from build123d import *

# Parameters (mm, degrees)
F0_W     = 31.75
F0_H     = 16.51
F0_W_2   = 26.67
F0_H_2   = 11.43
F1_DEPTH = 304.8
F2_SIZE  = 1.27
F3_SIZE  = 1.27
F5_D     = 12.7
F5_DEPTH = 25.4


with BuildPart() as f1:
    # F0 (on Top) → F1 (new body)
    with BuildSketch(Plane.XY):
        Rectangle(F0_W, F0_H)
        Rectangle(F0_W_2, F0_H_2, mode=Mode.SUBTRACT)
    extrude(amount=F1_DEPTH)

    # F2
    f2_edges = [f1.edges().sort_by_distance(p)[0] for p in [
        (0, 5.715, 304.8),
        (-13.335, 0, 304.8),
        (0, -5.715, 304.8),
        (13.335, 0, 304.8),
    ]]
    chamfer(f2_edges, length=F2_SIZE)

    # F3
    f3_edges = [f1.edges().sort_by_distance(p)[0] for p in [
        (13.335, 0, 0),
        (0, 5.715, 0),
        (-13.335, 0, 0),
        (0, -5.715, 0),
    ]]
    chamfer(f3_edges, length=F3_SIZE)

    # F5
    with Locations(Plane.XZ.offset(8.255)):
        with Locations((0, 152.39365), (0, 247.65), (0.458365, 57.15)):
            Hole(F5_D / 2, depth=F5_DEPTH)


solid = f1.part
The listing builds one solid part. Answer for the finished solid, in the listing's coordinates (mm). A direction names the side the tool comes from. Give positions to 0.01 mm unless a question says otherwise; leave off trailing zeros. Write each loop counter-clockwise with the first axis right and the second up, starting at its lowest first coordinate (ties: lowest second). Pieces come first, ordered by that corner, then holes. Notation, with made-up numbers: (-18.5, -32.5) - (36.5, -32.5) arc R12 cw to (36.5, -10.5) - close; hole circle Ø3 at (62.5, 74.5). An arc over 180 degrees is marked (long way). Use a Markdown table: item, result.
1. A tool of negligible diameter and unlimited length cuts with its end or side. For faces 1 (the flat face through (-9, 5.715, 150)), 2 (the cylindrical face through (1.38, 7, 241.45)), from which of +Z, -Z, +X, -X, +Y, -Y can it reach the whole face along a straight path? Write none if from no direction.
Values follow:
| item | result |
|---|---|
| face 1 | +Z, -Z |
| face 2 | +Y, -Y |
2. Section C-C on z = 79.5 is taken. Write down the section's boundary in (x, y) (3 decimals).
Values follow:
| item | result |
|---|---|
| outline | (-15.875, -8.255) - (15.875, -8.255) - (15.875, 8.255) - (-15.875, 8.255) - close; hole (-13.335, -5.715) - (13.335, -5.715) - (13.335, 5.715) - (-13.335, 5.715) - close |
3. For a pull along X with two mould halves and no side action, classify faces 3 (the flat face through (-1.3, -7.3, 0)), 4 (the flat face through (-9, -5.715, 150)), 5 (the flat face through (15.875, 0, 150)), 6 (the flat face through (-15.875, 0, 150)) as released by +X, released by -X, zero draft, split by the parting line, or undercut.
Values follow:
| item | result |
|---|---|
| face 3 | zero draft |
| face 4 | undercut |
| face 5 | released by +X |
| face 6 | released by -X |
4. Section D-D on x = 2 is taken. Count the separate pieces of the cut face and the enclosed holes in it, plus the area to 3 significant figures.
Values follow:
| item | result |
|---|---|
| separate pieces | 8 |
| enclosed holes | 0 |
| area | 1,360 mm² |
5. Section B-B on y = 0.5 is taken. Write down the section's boundary in (x, z) (3 decimals).
Values follow:
| item | result |
|---|---|
| outline | (-15.875, 0) - (-14.605, 0) - (-13.335, 1.27) - (-13.335, 303.53) - (-14.605, 304.8) - (-15.875, 304.8) - close; (13.335, 1.27) - (14.605, 0) - (15.875, 0) - (15.875, 304.8) - (14.605, 304.8) - (13.335, 303.53) - close |
6. Each of these flat-tipped pins is pushed along its axis until it touches: P1, Ø6, axis at x = -11, y = 2.5, coming from the +Z side (3 decimals); P2, Ø7.5, axis at x = 0, z = 152.39, coming from the -Y side. Where does it stop, or does it pass through?
Values follow:
| item | result |
|---|---|
| P1 | stops at z = 304.195 |
| P2 | passes through |
7. Find the intervals of material crossed by probe 1 along Z at (x, y) = (0, 7.3); probe 2 along X at (y, z) = (5, 288.5) (3 decimals); probe 3 along Y at (x, z) = (7, 263) (3 decimals), in increasing order. Write a range as from..to.
Values follow:
| item | result |
|---|---|
| probe 1 | z = 0..50.82, 63.48..146.04, 158.74..241.3, 254..304.8 |
| probe 2 | x = -15.875..-13.335, 13.335..15.875 |
| probe 3 | y = -8.255..-5.715, 5.715..8.255 |
8. Section A-A on z = 247.65 is taken. Write down the section's boundary in (x, y) (3 decimals).
Values follow:
| item | result |
|---|---|
| outline | (-15.875, -8.255) - (-6.35, -8.255) - (-6.35, -5.715) - (-13.335, -5.715) - (-13.335, 5.715) - (-6.35, 5.715) - (-6.35, 8.255) - (-15.875, 8.255) - close; (6.35, -8.255) - (15.875, -8.255) - (15.875, 8.255) - (6.35, 8.255) - (6.35, 5.715) - (13.335, 5.715) - (13.335, -5.715) - (6.35, -5.715) - close |
